Here's the drawing with two shaded views (mm, measured from the low corner). I have some questions. Give positions to 0.01 mm unless a question says otherwise; leave off trailing zeros. Write each loop counter-clockwise with the first axis right and the second up, starting at its lowest first coordinate (ties: lowest second). Pieces come first, ordered by that corner, then holes.
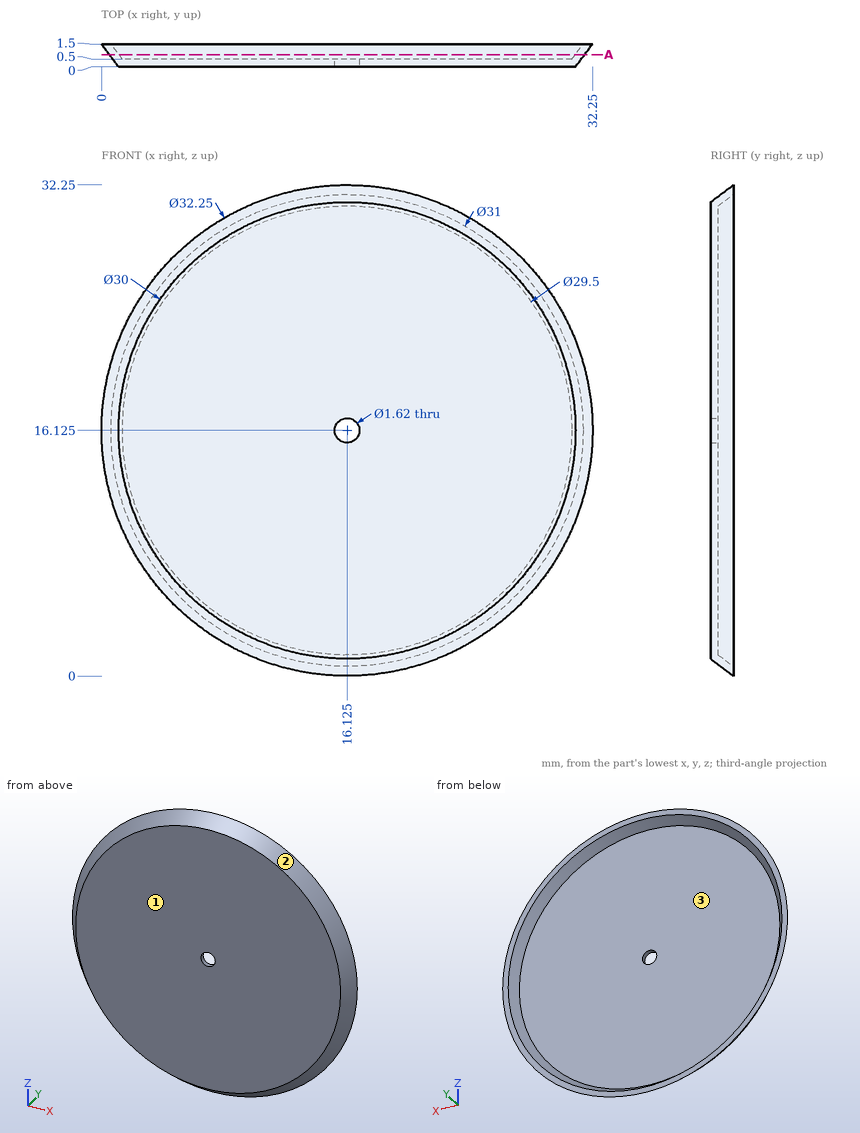
1) Please list where these lines run through material, in increasing order: L1, parallel to Y at x = 17, z = 25; L2, parallel to Z at x = 24, y = 1; L3, parallel to X at y = 1.25, z = 29.5.
Values follow:
L1: y = 0 to 0.5
L2: z = 2.49 to 3.21, 29.04 to 29.76
L3: x = 7.46 to 8.67, 23.58 to 24.79
2) For pin 1 Ø5 at (x, z) = (25.5, 25.5) entering from +Y; pin 2 Ø15 at (x, z) = (13, 20) entering from +Y, each with a flat end and sliding along its axis, tell me the tip position at first contact or that it passes through.
Values follow:
pin 1: stops at y = 1.5
pin 2: stops at y = 0.5
3) If we mould it in two halves opening along X, with no side actions, what happens to the marked faces 1, 2 and 3? For each: +X half, -X half, draft (parallel to the pull), parting line (faces both ways), or undercut.
Values follow:
face 1: draft
face 2: parting line
face 3: undercut
4) Suppose I cut it at A-A on y = 0.8. Write out the boundary of the cut face in (x, z) (3 decimals), plus the area to 3 significant figures.
Values follow:
outline: circle Ø31.2 at (16.125, 16.125); hole circle Ø29.95 at (16.125, 16.125)
area: 60.0 mm2
